Geometry: final body of the model. Coordinates: model frame, mm. Face numbers are marked on the shaded views. Coordinates: 2 decimals unless noted, no trailing zeros. Write each loop counter-clockwise with the first axis right and the second up, starting at its lowest first coordinate (ties: lowest second). Pieces come first, ordered by that corner, then holes. Notation, with made-up numbers: (67, 66) - (91, 66) arc R21 cw to (91, 71) - close; hole circle Ø8 at (66, 61.25). An arc over 180 degrees is marked (long way). Put each result on its own line as item: value.
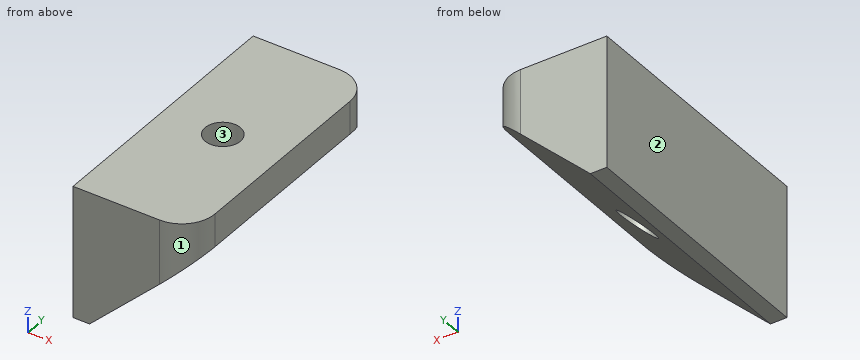
```python
from build123d import *

# Parameters (mm, degrees)
F0_W        = 22.987
F0_H        = 25.4
F1_DEPTH    = 25.4
F2_R        = 6.35
F4_D        = 6.8
F5_T1_DEPTH = 140.0532259942


# Not quite as in the source:
# - a fillet or chamfer that OpenCascade refuses, or shapes differently, is made with other operations: its cross-section is extruded or revolved along the edge and cut away or added


with BuildPart() as f1:
    # F0 (on Front) → F1 (new body, symmetric)
    with BuildSketch(Plane.XZ):
        Rectangle(F0_W, F0_H)
    extrude(amount=F1_DEPTH, both=True)

    # F2
    f2_edges = [f1.edges().sort_by_distance(p)[0] for p in [
        (11.4935, 25.4, 0),
        (11.4935, -25.4, 0),
    ]]
    fillet(f2_edges, radius=F2_R)

    # F4 (through all)
    with Locations(Plane.XY.offset(12.7)):
        with Locations((0, 0)):
            Hole(F4_D / 2)

    # F5: chamfer of 19.05 x 19.812 on 1 edges, made by hand

    # F5_s2 → F5_t1 (cut)
    with BuildSketch(Plane.XZ.offset(-70.0266129971)):
        Polygon((11.4935, 6.35), (-8.3185, -12.7), (11.4935, -12.7), align=None)
    extrude(amount=F5_T1_DEPTH, mode=Mode.SUBTRACT)


solid = f1.part
```
1. Section query D-D (z = 1.5). Return loops of the section in (x, y), then the cut area to 3 significant figures.
Answer below:
outline: (-11.49, -25.4) - (5.14, -25.4) arc R6.35 ccw to (6.45, -25.26) - (6.45, 25.26) arc R6.35 ccw to (5.14, 25.4) - (-11.49, 25.4) - close; hole circle Ø6.8 at (0, 0)
area: 875 mm²
2. Section query C-C (y = 0). Return loops of the section in (x, z).
Answer below:
outline: (-11.49, -12.7) - (-8.32, -12.7) - (-3.4, -7.97) - (-3.4, 12.7) - (-11.49, 12.7) - close; (3.4, -1.43) - (11.49, 6.35) - (11.49, 12.7) - (3.4, 12.7) - close
3. Section query A-A (z = 9.75). Return loops of the section in (x, y), then the cut area to 3 significant figures.
Answer below:
outline: (-11.49, -25.4) - (5.14, -25.4) arc R6.35 ccw to (11.49, -19.05) - (11.49, 19.05) arc R6.35 ccw to (5.14, 25.4) - (-11.49, 25.4) - close; hole circle Ø6.8 at (0, 0)
area: 1,110 mm²
4. Section query B-B (x = 0). Return loops of the section in (y, z).
Answer below:
outline: (-25.4, -4.7) - (-3.4, -4.7) - (-3.4, 12.7) - (-25.4, 12.7) - close; (3.4, -4.7) - (25.4, -4.7) - (25.4, 12.7) - (3.4, 12.7) - close
5. Ray query, probe 1 along Y at (x, z) = (0, 1.25); probe 2 along X at (y, z) = (0, 7.5); probe 3 along X at (y, z) = (0, 2.25). Return the intervals inside material, ascending. Write a range as from..to.
Answer below:
probe 1: y = -25.4..-3.4, 3.4..25.4
probe 2: x = -11.49..-3.4, 3.4..11.49
probe 3: x = -11.49..-3.4, 3.4..7.23
6. Mould query, pull axis Y, two halves, no side actions, for the marked faces 1, 2 and 3. Classes: +Y half, -Y half, draft (parallel to the pull), parting line (faces both ways), or undercut.
Answer below:
face 1: -Y half
face 2: draft
face 3: undercut
7. Pin query (flat end, axial travel): pin 1 Ø2 at (y, z) = (8, -0.5) entering from +X; pin 2 Ø8 at (x, y) = (0, 0) entering from -Z. Return the tip coordinate at first contact, or that it passes through.
Answer below:
pin 1: stops at x = 5.41
pin 2: stops at z = -8.55
